Could you check a few things on this drawing? It's one solid part, dimensions in mm from its lowest x, y, z. Give positions to 0.01 mm unless a question says otherwise; leave off trailing zeros. Order: outer loops, then holes, each group sorted by start corner. A loop starts at its lowest first (then second) coordinate and runs counter-clockwise, first axis right, second up.
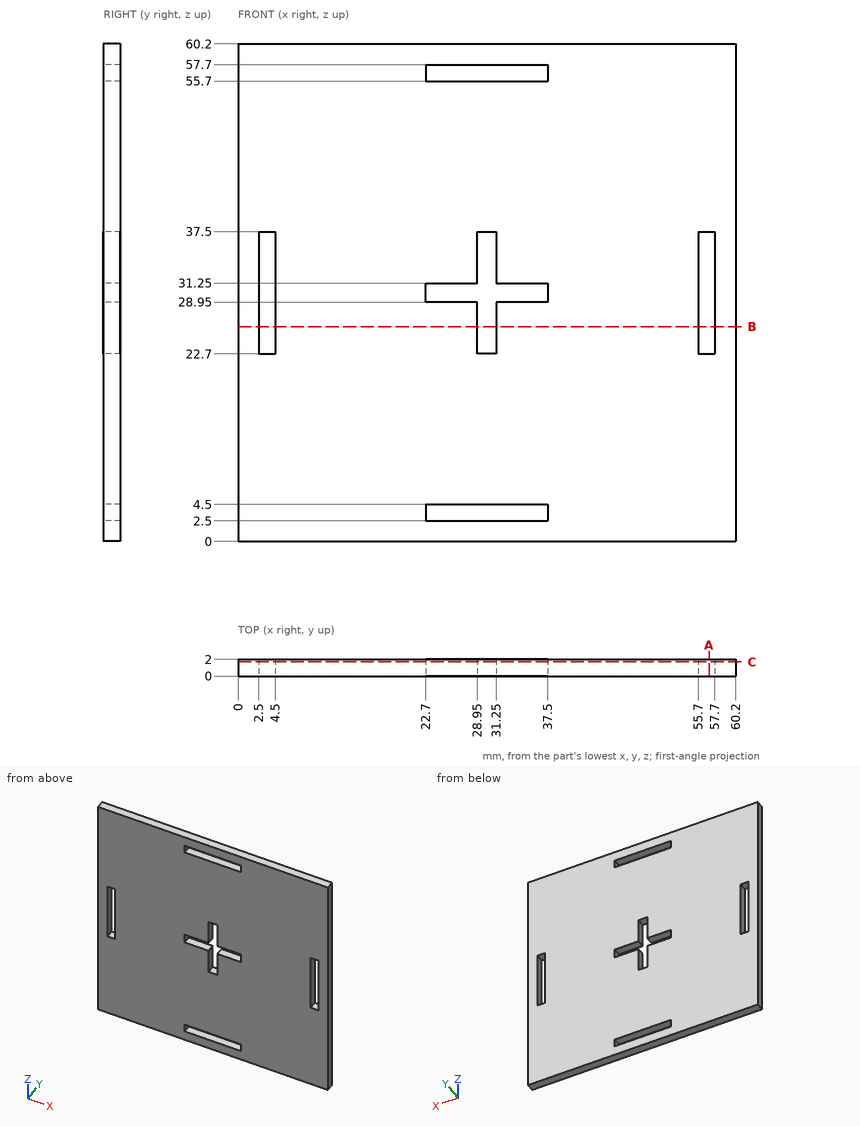
Q1. If we section it at B-B on z = 26: List the corners of the cut face in (x, y) for me, plus the area to 3 significant figures.
Filled sheet:
outline: (0, 0) - (2.5, 0) - (2.5, 2) - (0, 2) - close; (4.5, 0) - (28.95, 0) - (28.95, 2) - (4.5, 2) - close; (31.25, 0) - (55.7, 0) - (55.7, 2) - (31.25, 2) - close; (57.7, 0) - (60.2, 0) - (60.2, 2) - (57.7, 2) - close
area: 108 mm2
Q2. If we section it at A-A on x = 57: List the corners of the cut face in (y, z) for me, plus the area to 3 significant figures.
Filled sheet:
outline: (0, 0) - (2, 0) - (2, 22.7) - (0, 22.7) - close; (0, 37.5) - (2, 37.5) - (2, 60.2) - (0, 60.2) - close
area: 90.8 mm2
Q3. I need wall thicknesses on L1, parallel to Z at x = 23.5, y = 1.75; L2, parallel to Z at x = 4, y = 1.15. Which ranges of each line are inside material? Lowest first, please.
Filled sheet:
L1: z = 0 to 2.5, 4.5 to 28.95, 31.25 to 55.7, 57.7 to 60.2
L2: z = 0 to 22.7, 37.5 to 60.2
Q4. If we section it at C-C on y = 1.7: Give the number of separate pieces and of enclosed holes in the cut face, plus the area to 3 significant figures.
Filled sheet:
separate pieces: 1
enclosed holes: 5
area: 3,440 mm2
